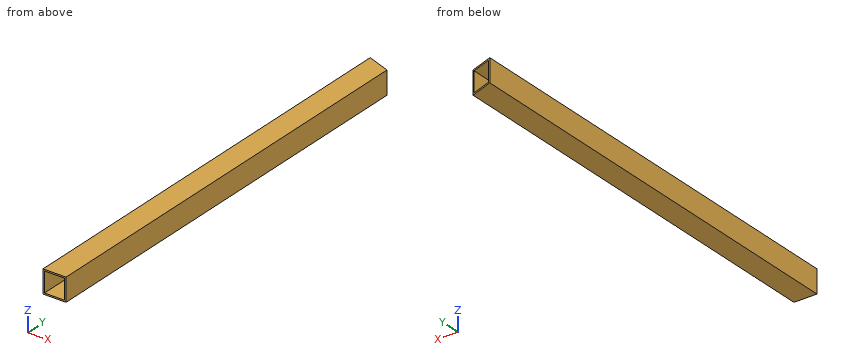
```python
from build123d import *

# Parameters (mm, degrees)
SKETCH1_W           = 25.4
SKETCH1_H           = 25.4
SKETCH1_W_2         = 22.225
SKETCH1_H_2         = 22.225
BOSS_EXTRUDE1_DEPTH = 482.6
CUT_EXTRUDE1_DEPTH  = 25.4


with BuildPart() as part:
    # Sketch1 → Boss-Extrude1 (new body)
    with BuildSketch(Plane(origin=(0, 0, 0), x_dir=(1, 0, 0), z_dir=(0, 1, 0))):
        Rectangle(SKETCH1_W, SKETCH1_H)
        Rectangle(SKETCH1_W_2, SKETCH1_H_2, mode=Mode.SUBTRACT)
    extrude(amount=BOSS_EXTRUDE1_DEPTH)

    # Sketch2 → Cut-Extrude1 (cut)
    with BuildSketch(Plane.XY.offset(12.7)):
        Polygon((-12.7, 482.6), (12.7, 473.35515605), (12.7, 482.6), align=None)
    extrude(amount=-CUT_EXTRUDE1_DEPTH, mode=Mode.SUBTRACT)


solid = part.part
```
Could you check a few things on this model? Use its own coordinates, in mm. Round coordinates to 2 decimals unless told otherwise and drop trailing zeros. Loops run counter-clockwise (first coordinate to the right, second up) from the corner with the lowest first, then second, coordinate; pieces in that order, holes last. Notation, with made-up numbers: (33, 57.5) - (91, 57.5) arc R27 cw to (91, 83.5) - close; hole circle Ø2 at (3.25, 84.25). An arc over 180 degrees is marked (long way). Use CSV: the item, a comma, the result in double quotes.
Item 1: Will these pins go through, and if not, where does the flat tip stop? pin 1 (5 mm diameter, centred on x = 3, z = -9, fed in from +Y); pin 2 (4 mm diameter, centred on x = 7.5, z = 10, fed in from +Y); pin 3 (12 mm diameter, centred on x = 9, z = -3.5, fed in from -Y).
Here are the results:
pin 1,"stops at y = 477.37"
pin 2,"stops at y = 475.85"
pin 3,"stops at y = 0"
Item 2: If we section it at A-A on z = 0.5: List the corners of the cut face in (x, y) for me, then the cut area to 3 significant figures.
Here are the results:
outline,"(-12.7, 0) - (-11.11, 0) - (-11.11, 482.02) - (-12.7, 482.6) - close; (11.11, 0) - (12.7, 0) - (12.7, 473.36) - (11.11, 473.93) - close"
area,"1,520 mm²"
Item 3: If we section it at C-C on x = 2.25: List the corners of the cut face in (y, z) for me.
Here are the results:
outline,"(0, -12.7) - (477.16, -12.7) - (477.16, -11.11) - (0, -11.11) - close; (0, 11.11) - (477.16, 11.11) - (477.16, 12.7) - (0, 12.7) - close"
Item 4: If we section it at B-B on y = 400: List the corners of the cut face in (x, z) for me, then the cut area to 3 significant figures.
Here are the results:
outline,"(-12.7, -12.7) - (12.7, -12.7) - (12.7, 12.7) - (-12.7, 12.7) - close; hole (-11.11, -11.11) - (11.11, -11.11) - (11.11, 11.11) - (-11.11, 11.11) - close"
area,"151 mm²"
Item 5: I need wall thicknesses on L1, parallel to X at y = 192.5, z = -3.25. Which ranges of the line are inside material? Lowest first, please. Write a range as [from, to].
Here are the results:
L1,"x = [-12.7, -11.11], [11.11, 12.7]"
